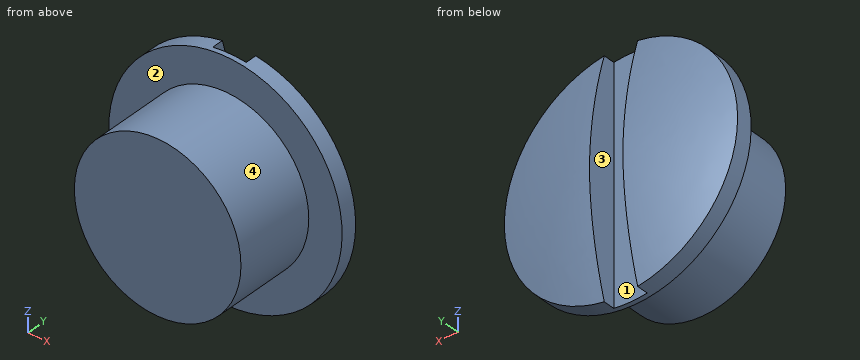
Autodesk Inventor part; units mm, degrees
ref_plane "Plano de trabalho1" through (0, 4.25, 0) normal (0, -1, 0) x (1, 0, 0)
ref_plane "YZ Plane" through (0, 0, 0) normal (1, 0, 0) x (0, 1, 0)
ref_plane "XZ Plane" through (0, 0, 0) normal (0, 1, 0) x (-1, 0, 0)
sketch "Esboço1" plane through (0, 0, 0) normal (1, 0, 0) x (0, 1, 0)
  line L0 (0, 0) -> (2.5, 0)
  line L1 (2.5, -2.5) -> (2.5, -3.5)
  line L2 (2.5, -3.5) -> (3, -3.5)
  line L3 (2.5, 0) -> (3, 0)
  line L4 (2.5, 0) -> (3.693, 0)
  arc A0 (3, -3.5) -> (3.564, 0) centre (-9.2697, 0.2726) ccw
  line L5 (0, 0) -> (0, -2.5)
  line L6 (0, -2.5) -> (2.5, -2.5)
  dimension "d0" = 2.5
  dimension "d1" = 3.5
  dimension "d3" = 0.5
  dimension "d11" = 2.5
revolve "Revolução1" add sketch "Esboço1" angle 360 about axis through (0, 0, 0) along (0, 1, 0)
thread "Rosca1"
ref_plane "Plano de trabalho1" through (0, 4.25, 0) normal (0, -1, 0) x (1, 0, 0)
sketch "Esboço2" plane through (0, 4.25, 0) normal (0, -1, 0) x (1, 0, 0)
  line L0 (-0.5012, 4.0955) -> (0.5012, 4.0955)
  line L1 (0.5012, 4.0955) -> (0.5012, -4.0955)
  line L2 (0.5012, -4.0955) -> (-0.5012, -4.0955)
  line L3 (-0.5012, -4.0955) -> (-0.5012, 4.0955)
  line L4 (-0.5012, 4.0955) -> (0.5012, -4.0955) construction
  line L5 (0.5012, 4.0955) -> (-0.5012, -4.0955) construction
  point P0 (0, 0)
extrude "Extrusão1" cut sketch "Esboço2" along normal blind 1.6
properties part number "parafusos"
CAD build for the part. Positions are in the model's coordinates, mm. Face numbers are marked on the shaded views. Round coordinates to 2 decimals unless told otherwise and drop trailing zeros. Order: outer loops, then holes, each group sorted by start corner. A loop starts at its lowest first (then second) coordinate and runs counter-clockwise, first axis right, second up.
Q1. Slice it at B-B (y = 1.05). Write the cut outline in (x, z), and give its area (3 significant figures).
Q2. Slice it at A-A (x = 0). Write the cut outline in (y, z), and give its area (4 significant figures).
Q3. Two-plate mould, pull along X, no slides. Class the marked faces 1, 2, 3 and 4: pulls with the +X half, pulls with the -X half, needs draft (parallel to the pull), parting line crosses it, or undercut.
Q4. Wall check: L1, parallel to Z at x = 0, y = 1.5; L2, parallel to Y at x = 0.25, z = -0.5. Give the ranges that are in metal, low to high.
Q5. Drop flat-ended pins along their axis: pin 1 (0.7 mm diameter, centred on y = 3, z = 1, fed in from +X); pin 2 (1.5 mm diameter, centred on y = 1, z = 1, fed in from +X); pin 3 (0.5 mm diameter, centred on x = 0, z = 0.5, fed in from +Y). Give the stop position or say it passes through.
Results below:
1. outline: circle Ø5 at (0, 0)
1. area: 19.6 mm2
2. outline: (0, -2.5) - (2.5, -2.5) - (2.5, -3.5) - (2.65, -3.5) - (2.65, 3.5) - (2.5, 3.5) - (2.5, 2.5) - (0, 2.5) - close
2. area: 13.55 mm2
3. face 1: undercut
3. face 2: needs draft
3. face 3: undercut
3. face 4: parting line crosses it
4. L1: z = -2.5 to 2.5
4. L2: y = 0 to 2.65
5. pin 1: stops at x = 3.44
5. pin 2: stops at x = 2.49
5. pin 3: stops at y = 2.65
